Can you work these out from the model? Positions are in its coordinate system, mm. A direction names the side the tool comes from. Round coordinates to 2 decimals unless told otherwise and drop trailing zeros. Write each loop counter-clockwise with the first axis right and the second up, starting at its lowest first coordinate (ties: lowest second). Pieces come first, ordered by that corner, then holes. Notation, with made-up numbers: M 55.5,54.5 L 108.5,54.5 A27 cw 108.5,77.5 Z; hole C 14.5,14 d9. An arc over 180 degrees is marked long. Answer in a Markdown table with one row per item. Add a question column.
(1) For faces 1 (the face through (-11.799, 2.442, 0.201)), 2 (the face through (0.2, -23.71, 0.2)), 3 (the face through (8.742, -22.596, 1.997)), 4 (the face through (29, -2, 0.864)), which set-ups out of +Z, -Z, +X, -X, +Y, -Y let a thin tool reach every point of the face, with its end or its side?
(2) Suppose I cut it at C-C, the plane y = 2.5. Write out the boundary of the cut face in (x, z), then the cut area to 3 significant figures.
(3) Suppose I cut it at A-A, the plane y = -15. Write out the boundary of the cut face in (x, z), then the cut area to 3 significant figures.
(4) If I drill on probe 1 along Y at (x, z) = (15.5, 1.4); probe 2 along X at (y, z) = (-2, 3.6); probe 3 along Y at (x, z) = (-0.5, 1.5), over which ranges is the centre line in solid material (lowest first)?
(5) I'm going to push flat-ended pins straight in: pin 1 (1 mm diameter, centred on x = 26, z = 2.5, fed in from +Y); pin 2 (2 mm diameter, centred on x = 17.5, y = -2, fed in from +Z); pin 3 (1.9 mm diameter, centred on y = -6.5, z = 1, fed in from +X); pin 4 (0.7 mm diameter, centred on y = -31, z = 2, fed in from -X). Where does each tip first touch, or does it pass through?
(6) Suppose I cut it at B-B, the plane x = 5. Write out the boundary of the cut face in (y, z).
(7) If we mould it in two halves opening along X, with no side actions, what happens to faces 5 (the face through (13.3, -18.9, 4.039)), 6 (the face through (5.81, -3.86, 3.84)), 7 (the face through (-16.2, 10.32, 3.43)), 8 (the face through (32.286, -37.606, 2.932))? For each: released by +X, released by -X, zero draft, split by the parting line, or undercut.
(8) Suppose I cut it at D-D, the plane x = -7. Write out the boundary of the cut face in (y, z).
from build123d import *

# Parameters (mm, degrees)
F15_DEPTH = 2.8194
F1_W      = 50.4952
F1_H      = 50.038
F2_DEPTH  = 1.2192
F3_R      = 1.016
F4_DEPTH  = 3.175
F5_W      = 25.5439807123
F5_H      = 7.9756
F6_DEPTH  = 4.0396
F7_W      = 10.16
F7_H      = 12.3698
F8_DEPTH  = 2.032
F9_R      = 3.81
F10_R     = 3.175
F11_R     = 1.5875
F12_SIZE  = 0.396875
F13_SIZE  = 0.396875


# Not quite as in the source:
# - a feature of the source that left no trace in its solid (it failed there, or was rolled back) is left out


with BuildPart() as f15:
    # F0 (on Top) → F15 (new body)
    with BuildSketch(Plane.XY):
        Polygon((30.4991698359, 9.5009198412), (-14.2048301641, 9.5009198412), (-14.2048301641, 5.0559198412), (-8.8708301641, -1.4210801588), (-2.8619992453, 1.1873513896), (2.9147698359, -5.378930905), (8.8075698359, -2.7315337496), (14.7003698359, -9.3367816513), (21.6091698359, -9.3367816513), (21.6091698359, -16.3653786662), (14.7003698359, -16.3653786662), (8.8075698359, -22.970626568), (2.9147698359, -20.3232294125), (-2.8619992453, -26.8895117072), (-8.8708301641, -24.2810801588), (-14.2048301641, -30.7580801588), (-14.2048301641, -35.2030801588), (30.4991698359, -35.2030801588), align=None)
    extrude(amount=F15_DEPTH)

    # F1 (on face) → F2 (join)
    with BuildSketch(Plane.XY.offset(2.8194)):
        with Locations((8.1471698359, -13.7400801588)):
            Rectangle(F1_W, F1_H)
        Polygon((-8.8708301641, -24.2810801588), (-14.2048301641, -30.7580801588), (-14.2048301641, 5.0559198412), (-8.8708301641, -1.4210801588), (-2.8619992453, 1.1873513896), (2.9147698359, -5.378930905), (8.8075698359, -2.7315337496), (14.7003698359, -9.3367816513), (21.6091698359, -9.3367816513), (21.6091698359, -16.3653786662), (14.7003698359, -16.3653786662), (8.8075698359, -22.970626568), (2.9147698359, -20.3232294125), (-2.8619992453, -26.8895117072), align=None, mode=Mode.SUBTRACT)
    extrude(amount=F2_DEPTH)

    # F3 (on face) → F4 (cut)
    with BuildSketch(Plane.XY.offset(4.0386)):
        with Locations((29.2672698359, -1.8401801588)):
            Circle(F3_R)
        with Locations((29.2672698359, -23.5825801588)):
            Circle(F3_R)
        with Locations((17.0752698359, -1.8401801588)):
            Circle(F3_R)
        with Locations((17.0752698359, -23.5825801588)):
            Circle(F3_R)
    extrude(amount=-F4_DEPTH, mode=Mode.SUBTRACT)

    # F5 (on face) → F6 (cut, through all)
    with BuildSketch(Plane(origin=(0, 0, 0), x_dir=(1, 0, 0), z_dir=(0, 0, -1))):
        with Locations((8.8371794797, 12.8510801588)):
            Rectangle(F5_W, F5_H)
    extrude(amount=-F6_DEPTH, mode=Mode.SUBTRACT)

    # F7 (on face) → F8 (cut)
    with BuildSketch(Plane.XY.offset(4.0386)):
        with Locations((26.6891698359, -10.6539801588)):
            Rectangle(F7_W, F7_H)
    extrude(amount=-F8_DEPTH, mode=Mode.SUBTRACT)

    # F9
    f9_edges = [f15.edges().sort_by_distance(p)[0] for p in [
        (-14.20483, -35.20308, 1.4097),
        (30.49917, -35.20308, 1.4097),
        (30.49917, 9.50092, 1.4097),
        (-14.20483, 9.50092, 1.4097),
    ]]
    fillet(f9_edges, radius=F9_R)

    # F10
    f10_edges = [f15.edges().sort_by_distance(p)[0] for p in [
        (33.39477, -38.75908, 3.429),
        (33.39477, 11.27892, 3.429),
        (-17.10043, 11.27892, 3.429),
        (-17.10043, -38.75908, 3.429),
    ]]
    fillet(f10_edges, radius=F10_R)

    # F11
    f11_edges = [f15.edges().sort_by_distance(p)[0] for p in [
        (-8.87083, -24.28108, 2.0193),
        (2.91477, -20.323229, 2.0193),
        (14.277941, -16.83888, 2.0193),
        (14.277941, -8.86328, 2.0193),
        (8.80757, -2.731534, 2.0193),
        (-2.861999, 1.187351, 2.0193),
        (-8.87083, -1.42108, 2.0193),
        (2.91477, -5.378931, 2.0193),
        (-2.861999, -26.889512, 2.0193),
        (8.80757, -22.970627, 2.0193),
    ]]
    fillet(f11_edges, radius=F11_R)

    # F12
    f12_edges = [f15.edges().sort_by_distance(p)[0] for p in [
        (-11.918021, -27.98124, 0),
        (-8.777201, -24.670149, 0),
        (-14.20483, -31.07558, 0),
        (-5.848035, -25.593275, 0),
        (-13.088907, -34.087157, 0),
        (-2.944073, -26.522248, 0),
        (8.14717, -35.20308, 0),
        (0.021273, -23.612182, 0),
        (29.383247, -34.087157, 0),
        (2.996452, -20.69995, 0),
        (30.49917, -12.85108, 0),
        (5.865037, -21.648665, 0),
        (29.383247, 8.384997, 0),
        (8.728242, -22.598537, 0),
        (8.14717, 9.50092, 0),
        (11.693168, -19.736155, 0),
        (-13.088907, 8.384997, 0),
        (14.340089, -16.97761, 0),
        (-14.20483, 5.37342, 0),
        (18.299137, -16.83888, 0),
        (-11.918021, 2.27908, 0),
        (21.60917, -12.85108, 0),
        (-8.777201, -1.032011, 0),
        (18.299137, -8.86328, 0),
        (-5.848035, -0.108886, 0),
        (14.340089, -8.72455, 0),
        (-2.944073, 0.820088, 0),
        (11.693168, -5.966005, 0),
        (0.021273, -2.089978, 0),
        (8.728242, -3.103623, 0),
        (2.996452, -5.00221, 0),
        (5.865037, -4.053495, 0),
    ]]
    chamfer(f12_edges, length=F12_SIZE)

    # F13
    f13_edges = [f15.edges().sort_by_distance(p)[0] for p in [
        (-14.20483, -12.85108, 2.8194),
        (-17.10043, -13.74008, 2.8194),
        (8.14717, -38.75908, 2.8194),
        (33.39477, -13.74008, 2.8194),
        (8.14717, 11.27892, 2.8194),
        (23.379137, -16.83888, 4.0386),
        (14.340089, -16.97761, 4.0386),
        (31.76917, -10.65398, 4.0386),
        (11.693168, -19.736155, 4.0386),
        (26.68917, -4.46908, 4.0386),
        (8.728242, -22.598537, 4.0386),
        (21.60917, -6.66618, 4.0386),
        (5.865037, -21.648665, 4.0386),
        (18.299137, -8.86328, 4.0386),
        (2.996452, -20.69995, 4.0386),
        (14.340089, -8.72455, 4.0386),
        (0.021273, -23.612182, 4.0386),
        (11.693168, -5.966005, 4.0386),
        (-2.944073, -26.522248, 4.0386),
        (8.728242, -3.103623, 4.0386),
        (-5.848035, -25.593275, 4.0386),
        (5.865037, -4.053495, 4.0386),
        (-8.777201, -24.670149, 4.0386),
        (2.996452, -5.00221, 4.0386),
        (-11.918021, -27.98124, 4.0386),
        (0.021273, -2.089978, 4.0386),
        (-14.20483, -12.85108, 4.0386),
        (-2.944073, 0.820088, 4.0386),
        (-11.918021, 2.27908, 4.0386),
        (-5.848035, -0.108886, 4.0386),
        (-8.777201, -1.032011, 4.0386),
        (-17.10043, -13.74008, 4.0386),
        (-16.170494, 10.348984, 4.0386),
        (-16.170494, -37.829144, 4.0386),
        (8.14717, 11.27892, 4.0386),
        (8.14717, -38.75908, 4.0386),
        (32.464834, 10.348984, 4.0386),
        (32.464834, -37.829144, 4.0386),
        (33.39477, -13.74008, 4.0386),
        (16.05927, -23.58258, 4.0386),
        (28.25127, -23.58258, 4.0386),
        (16.05927, -1.84018, 4.0386),
        (28.25127, -1.84018, 4.0386),
        (-16.170494, 10.348984, 2.8194),
        (-16.170494, -37.829144, 2.8194),
        (32.464834, 10.348984, 2.8194),
        (32.464834, -37.829144, 2.8194),
    ]]
    chamfer(f13_edges, length=F13_SIZE)


solid = f15.part
Calculated:
| question | item | result |
|---|---|---|
| 1 | face 1 | -Z, -X |
| 1 | face 2 | -Z |
| 1 | face 3 | +Z, -Z |
| 1 | face 4 | +Z |
| 2 | outline | M -17.1,3.22 L -16.7,2.82 L -14.6,2.82 L -14.2,3.22 L -14.2,3.64 L -14.6,4.04 L -16.7,4.04 L -17.1,3.64 Z; M -12.1,0.4 L -11.59,0 L 30.1,0 L 30.5,0.4 L 30.5,2.82 L 33,2.82 L 33.39,3.22 L 33.39,3.64 L 33,4.04 L -11.59,4.04 L -12.1,3.64 Z |
| 2 | area | 178 mm² |
| 3 | outline | M -17.1,3.22 L -16.7,2.82 L -14.6,2.82 L -14.2,3.22 L -14.2,3.64 L -14.6,4.04 L -16.7,4.04 L -17.1,3.64 Z; M 21.61,0.4 L 22.01,0 L 30.1,0 L 30.5,0.4 L 30.5,2.01 L 21.61,2.01 Z; M 31.77,2.82 L 33,2.82 L 33.39,3.22 L 33.39,3.64 L 33,4.04 L 32.17,4.04 L 31.77,3.64 Z |
| 3 | area | 22.6 mm² |
| 4 | probe 1 | -35.2 to -16.84, -8.86 to 9.5 |
| 4 | probe 2 | -17.1 to -14.2, -0.06 to 16.07, 18.08 to 28.26, 30.27 to 33.39 |
| 4 | probe 3 | -35.2 to -24.2, -1.5 to 9.5 |
| 5 | pin 1 | y = 11.06 |
| 5 | pin 2 | z = 4.04 |
| 5 | pin 3 | x = 30.5 |
| 5 | pin 4 | x = -14.2 |
| 6 | outline | M -38.76,3.22 L -38.36,2.82 L -35.2,2.82 L -35.2,0.4 L -34.81,0 L -21.7,0 L -21.26,0.4 L -21.26,3.64 L -21.7,4.04 L -38.36,4.04 L -38.76,3.64 Z; M -4.44,0.4 L -4.01,0 L 9.1,0 L 9.5,0.4 L 9.5,2.82 L 10.88,2.82 L 11.28,3.22 L 11.28,3.64 L 10.88,4.04 L -4.01,4.04 L -4.44,3.64 Z |
| 7 | face 5 | zero draft |
| 7 | face 6 | undercut |
| 7 | face 7 | released by -X |
| 7 | face 8 | released by +X |
| 8 | outline | M -38.76,3.22 L -38.36,2.82 L -35.2,2.82 L -35.2,0.4 L -34.81,0 L -25.53,0 L -25.09,0.4 L -25.09,3.64 L -25.53,4.04 L -38.36,4.04 L -38.76,3.64 Z; M -0.61,0.4 L -0.18,0 L 9.1,0 L 9.5,0.4 L 9.5,2.82 L 10.88,2.82 L 11.28,3.22 L 11.28,3.64 L 10.88,4.04 L -0.18,4.04 L -0.61,3.64 Z |
